Autodesk Inventor part; units mm, degrees
ref_plane "YZ Plane" through (0, 0, 0) normal (1, 0, 0) x (0, 1, 0)
ref_plane "XZ Plane" through (0, 0, 0) normal (0, 1, 0) x (-1, 0, 0)
ref_plane "XY Plane" through (0, 0, 0) normal (0, 0, 1) x (1, 0, 0)
sketch "スケッチ1" plane through (0, 0, 0) normal (1, 0, 0) x (0, 1, 0)
  line L0 (-12.5, 12.5) -> (12.5, 12.5)
  line L1 (12.5, 12.5) -> (12.5, -12.5)
  line L2 (12.5, -12.5) -> (-12.5, -12.5)
  line L3 (-12.5, -12.5) -> (-12.5, 12.5)
  line L4 (-12.5, 12.5) -> (12.5, -12.5) construction
  line L5 (12.5, 12.5) -> (-12.5, -12.5) construction
  point P0 (0, 0)
  dimension "d0" = 25
  dimension "d1" = 25
extrude "押し出し1" add sketch "スケッチ1" along normal blind 55
sketch "スケッチ2" plane through (0, 12.5, 12.5) normal (0, 1, 0) x (1, 0, 0)
  circle A0 centre (10, 12.5) radius 6
  line L0 (0, 0) -> (0, 25)
  line L1 (0, 0) -> (55, 0)
  point P0 (0, 12.5)
  dimension "d4" = 12
  dimension "d5" = 10
  dimension "d6" = 12.5
extrude "押し出し2" cut sketch "スケッチ2" against normal through all
sketch "スケッチ3" plane through (0, 12.5, 12.5) normal (0, 1, 0) x (1, 0, 0)
  circle A0 centre (45, 12.5) radius 4
  line L0 (55, 25) -> (55, 0)
  line L1 (0, 25) -> (55, 25)
  point P0 (0, 12.5)
  dimension "d9" = 10
  dimension "d10" = 8
  dimension "d11" = 12.5
extrude "押し出し3" cut sketch "スケッチ3" against normal through all
sketch "スケッチ4" plane through (55, 0, 0) normal (1, 0, 0) x (0, 0, -1)
  line L0 (-10.2, -10.2) -> (10.2, -10.2)
  line L1 (10.2, -10.2) -> (10.2, 10.2)
  line L2 (10.2, 10.2) -> (-10.2, 10.2)
  line L3 (-10.2, 10.2) -> (-10.2, -10.2)
  line L4 (-10.2, -10.2) -> (10.2, 10.2) construction
  line L5 (10.2, -10.2) -> (-10.2, 10.2) construction
  line L6 (-12.5, 12.5) -> (-12.5, -12.5)
  line L7 (12.5, 12.5) -> (-12.5, 12.5)
  point P0 (0, 0)
  dimension "d14" = 2.3
  dimension "d15" = 2.3
extrude "押し出し4" cut sketch "スケッチ4" against normal through all
sketch "スケッチ5" plane through (0, -12.5, -12.5) normal (0, 0, -1) x (-1, 0, 0)
  line L0 (-55, 2.3) -> (-55, 22.7)
  line L1 (-55, 2.3) -> (0, 2.3)
  line L2 (-55, 22.7) -> (-35, 22.7)
  line L3 (-35, 22.7) -> (-35, 2.3)
  line L4 (-35, 2.3) -> (-55, 2.3)
  line L5 (-55, 2.3) -> (-55, 22.7)
  point P0 (0, 12.5)
  dimension "d18" = 20
extrude "押し出し5" cut sketch "スケッチ5" against normal through all
fillet "フィレット1" radius 7 8 edges at (55, 11.35, -12.5) (55, -11.35, -12.5) (55, -11.35, 12.5) (55, 11.35, 12.5) (35, -10.2, -11.35) (35, -10.2, 11.35) (35, 10.2, -11.35) (35, 10.2, 11.35)
equation "\"d1\" = d0"
properties part number "bracket FU RL" material "鉄、可鍛鉄"
Geometry: final body of the model. Coordinates: model frame, mm. A direction names the side the tool comes from. Coordinates: 2 decimals unless noted, no trailing zeros. Write each loop counter-clockwise with the first axis right and the second up, starting at its lowest first coordinate (ties: lowest second). Pieces come first, ordered by that corner, then holes. Notation, with made-up numbers: (26, -20) - (84, -20) arc R29 ccw to (84, 6) - close; hole circle Ø4 at (14, 10). An arc over 180 degrees is marked (long way). Return JSON: item names as keys, results as strings.
Item 1: Section query D-D (x = 45). Output: boundary loops of the cut face in (y, z).
Completed:
{"outline": "(-12.5, -12.5) - (-10.2, -12.5) - (-10.2, -4) - (-12.5, -4) - close; (-12.5, 4) - (-10.2, 4) - (-10.2, 12.5) - (-12.5, 12.5) - close; (10.2, -12.5) - (12.5, -12.5) - (12.5, -4) - (10.2, -4) - close; (10.2, 4) - (12.5, 4) - (12.5, 12.5) - (10.2, 12.5) - close"}
Item 2: Reachability of faces 5 (the face through (17, 0, -10.2)), 6 (the face through (37.1, 8.2, -11.3)), 7 (the face through (52.9, -11.4, -10.5)) from +Z, -Z, +X, -X, +Y, -Y: full face, straight path, thin tool, end or side. Return the list, or none.
Completed:
{"face 5": "+X, -X", "face 6": "+Z, -Z, +X", "face 7": "-Z, +X, +Y, -Y"}
Item 3: Section query A-A (x = 10). Output: boundary loops of the cut face in (y, z), and give its area (3 significant figures).
Completed:
{"outline": "(-12.5, -12.5) - (12.5, -12.5) - (12.5, -6) - (10.2, -6) - (10.2, -10.2) - (-10.2, -10.2) - (-10.2, -6) - (-12.5, -6) - close; (-12.5, 6) - (-10.2, 6) - (-10.2, 10.2) - (10.2, 10.2) - (10.2, 6) - (12.5, 6) - (12.5, 12.5) - (-12.5, 12.5) - close", "area": "154 mm2"}
Item 4: Pin query (flat end, axial travel): pin 1 Ø2.5 at (y, z) = (-0.5, -12) entering from +X; pin 2 Ø9.5 at (x, z) = (10, 0) entering from +Y. Return the tip coordinate at first contact, or that it passes through.
Completed:
{"pin 1": "stops at x = 35", "pin 2": "passes through"}
Item 5: Pull-direction query (Y, two-part tool) for faces 1 (the face through (28, 10.2, 0)), 2 (the face through (27, 12.5, 0)), 3 (the face through (55, 11, 0)), 4 (the face through (27, -12.5, 0)); classes: +Y half, -Y half, draft (parallel to the pull), parting line (faces both ways), or undercut.
Completed:
{"face 1": "undercut", "face 2": "+Y half", "face 3": "draft", "face 4": "-Y half"}
Item 6: Section query B-B (z = 0). Output: boundary loops of the cut face in (x, y).
Completed:
{"outline": "(0, -12.5) - (4, -12.5) - (4, -10.2) - (0, -10.2) - close; (0, 10.2) - (4, 10.2) - (4, 12.5) - (0, 12.5) - close; (16, -12.5) - (41, -12.5) - (41, -10.2) - (16, -10.2) - close; (16, 10.2) - (41, 10.2) - (41, 12.5) - (16, 12.5) - close; (49, -12.5) - (55, -12.5) - (55, -10.2) - (49, -10.2) - close; (49, 10.2) - (55, 10.2) - (55, 12.5) - (49, 12.5) - close"}
Item 7: Line query: L1, parallel to X at y = -11.6, z = 0; L2, parallel to Z at x = 10, y = -11.05; L3, parallel to Z at x = 21.5, y = -1.5. Output: solid intervals per line, ascending.
Completed:
{"L1": "x = 0 to 4, 16 to 41, 49 to 55", "L2": "z = -12.5 to -6, 6 to 12.5", "L3": "z = -12.5 to -10.2, 10.2 to 12.5"}
Item 8: Section query C-C (z = 8.25). Output: boundary loops of the cut face in (x, y).
Completed:
{"outline": "(0, -12.5) - (54.44, -12.5) - (54.44, -10.2) - (0, -10.2) - close; (0, 10.2) - (54.44, 10.2) - (54.44, 12.5) - (0, 12.5) - close"}
